Print and shaded views of the part. All mm, measured from the part's lowest x, y and z. A direction names the side the tool comes from. Coordinates: 2 decimals unless noted, no trailing zeros. Order: outer loops, then holes, each group sorted by start corner. A loop starts at its lowest first (then second) coordinate and runs counter-clockwise, first axis right, second up. Notation, with made-up numbers: M 72,-11 L 106,-11 A21 cw 106,7 Z; hole C 45.5,-17.5 d7. An arc over 180 degrees is marked long. One line per item, written item: value.
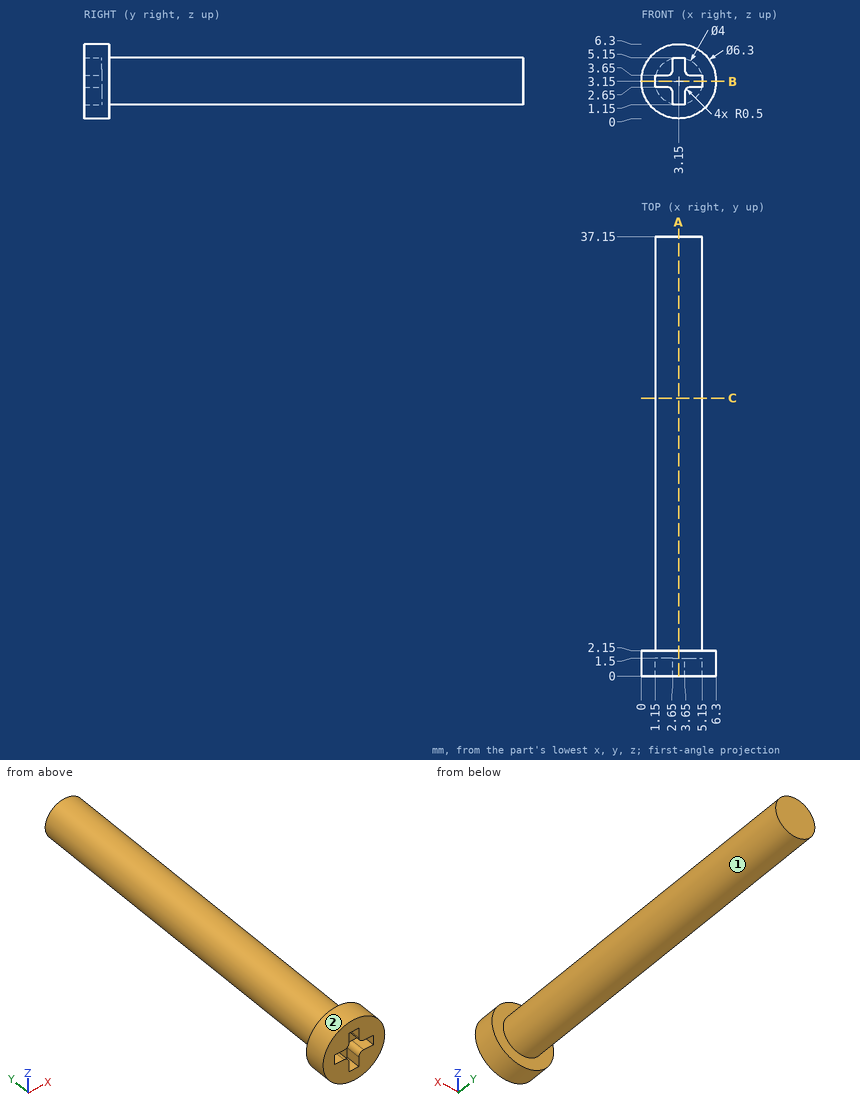
Q1. Slice it at C-C (y = 23.5). List the corners of the cut face in (x, z), plus the area to 3 significant figures.
Recorded:
outline: C 3.15,3.15 d4
area: 12.6 mm^2
Q2. Drill centre lines: line 1 along Y through (x, z) = (1.5, 5); line 2 along Y through (x, z) = (3, 2.5); line 3 along Z through (x, y) = (2.25, 18). Where is each one in solid material? Low to high.
Recorded:
line 1: y = 0 to 2.15
line 2: y = 1.5 to 37.15
line 3: z = 1.36 to 4.94
Q3. Slice it at A-A (x = 3.15). List the corners of the cut face in (y, z).
Recorded:
outline: M 0,0 L 2.15,0 L 2.15,1.15 L 37.15,1.15 L 37.15,5.15 L 2.15,5.15 L 2.15,6.3 L 0,6.3 L 0,5.15 L 1.5,5.15 L 1.5,1.15 L 0,1.15 Z
Q4. Pin check, flat tips, straight feed: pin 1 Ø1.1 at (y, z) = (1, 3) entering from +X; pin 2 Ø1.1 at (x, y) = (5, 1) entering from +Z; pin 3 Ø0.5 at (y, z) = (0.5, 1.5) entering from -X; pin 4 Ø0.5 at (y, z) = (1, 4.5) entering from +X. Stop position of each tip, or through.
Recorded:
pin 1: stops at x = 6.3
pin 2: stops at z = 6.02
pin 3: stops at x = 0.33
pin 4: stops at x = 6.1
Q5. Slice it at B-B (z = 3.15). List the corners of the cut face in (x, y), plus the area to 3 significant figures.
Recorded:
outline: M 0,0 L 1.15,0 L 1.15,1.5 L 5.15,1.5 L 5.15,0 L 6.3,0 L 6.3,2.15 L 5.15,2.15 L 5.15,37.15 L 1.15,37.15 L 1.15,2.15 L 0,2.15 Z
area: 148 mm^2
Q6. Which spindle directions (+Z, -Z, +X, -X, +Y, -Y) get a long thin tool onto all of the face, cutting with end or side? Do the marked faces 1 and 2. Say none if no direction does.
Recorded:
face 1: +Y
face 2: +Y, -Y
